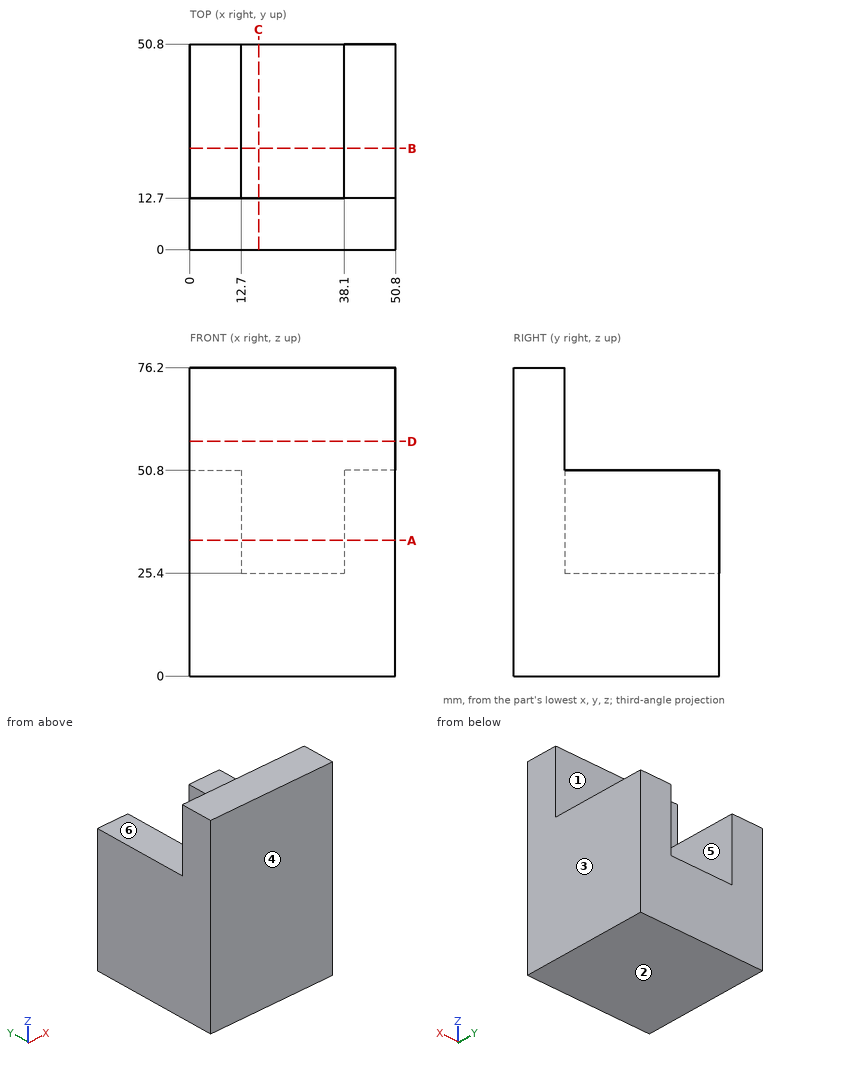
Study the drawing (mm; zero at the part's minimum x, y, z) and answer. A direction names the side the tool comes from. Give positions to 0.01 mm unless a question says otherwise; leave off trailing zeros. Write each loop counter-clockwise with the first axis right and the second up, starting at its lowest first coordinate (ties: lowest second). Pieces come first, ordered by that corner, then holes. Notation, with made-up numbers: (15, 60) -> (29, 60) arc R22 cw to (29, 79) -> close; hole circle Ø4 at (-10.5, -37.5). An arc over 180 degrees is marked (long way). Write item = value, one per line. Start each with the question number.
1) Which of the six approach directions +Z, -Z, +X, -X, +Y, -Y give full straight-line access (tool end or side, diameter ignored) to the marked faces 4, 5 and 6?
2) Straight lines are drawn through the part: line 1 along Y through (x, z) = (7, 72); line 2 along Z through (x, y) = (4.5, 27); line 3 along Z through (x, y) = (22, 23.5). For each, find the intervals that lie inside material, in ascending order.
3) The part is cut by section B-B, the plane y = 25. Determine the outline of the cut face in (x, z).
4) The part is cut by section A-A, the plane z = 33.5. Determine the outline of the cut face in (x, y), and give its area (3 significant figures).
5) Each of these flat-tipped pins is pushed along its axis until it touches: pin 1 (4 mm diameter, centred on x = 47, y = 29.5, fed in from +Z); pin 2 (7.5 mm diameter, centred on x = 31, y = 36, fed in from +Z); pin 3 (2 mm diameter, centred on x = 25.5, z = 60, fed in from +Y). Where does it stop, or does it pass through?
6) The part is cut by section C-C, the plane x = 17. Determine the outline of the cut face in (y, z), and give its area (3 significant figures).
7) The part is cut by section D-D, the plane z = 58. Determine the outline of the cut face in (x, y), and give its area (3 significant figures).
8) Determine the mould class of the marked faces 1, 2 and 3 for opening direction X: +X half, -X half, draft (parallel to the pull), parting line (faces both ways), or undercut.
Solutions:
q1.face_4 = +Z, -Z, +X, -X, -Y
q1.face_5 = +Z, +Y
q1.face_6 = +Z, +X, -X, +Y
q2.line_1 = 0 to 12.7
q2.line_2 = 0 to 50.8
q2.line_3 = 0 to 25.4
q3.outline = (0, 0) -> (50.8, 0) -> (50.8, 50.8) -> (38.1, 50.8) -> (38.1, 25.4) -> (12.7, 25.4) -> (12.7, 50.8) -> (0, 50.8) -> close
q4.outline = (0, 0) -> (50.8, 0) -> (50.8, 50.8) -> (38.1, 50.8) -> (38.1, 12.7) -> (12.7, 12.7) -> (12.7, 50.8) -> (0, 50.8) -> close
q4.area = 1,610 mm²
q5.pin_1 = 50.8
q5.pin_2 = 25.4
q5.pin_3 = 12.7
q6.outline = (0, 0) -> (50.8, 0) -> (50.8, 25.4) -> (12.7, 25.4) -> (12.7, 76.2) -> (0, 76.2) -> close
q6.area = 1,940 mm²
q7.outline = (0, 0) -> (50.8, 0) -> (50.8, 12.7) -> (0, 12.7) -> close
q7.area = 645 mm²
q8.face_1 = undercut
q8.face_2 = draft
q8.face_3 = +X half
